Work out the finished part from the listing and answer in its coordinate system (mm). Coordinates: 2 decimals unless noted, no trailing zeros. Order: outer loops, then holes, each group sorted by start corner. A loop starts at its lowest first (then second) coordinate and runs counter-clockwise, first axis right, second up. Notation, with made-up numbers: M -39,82 L -30,82 A19 cw -30,95 Z; hole C 74.5,-27 d3. An arc over 180 degrees is marked long. Answer in a Markdown table with one row per item. Add a question column.
Item 1: Consider line 1 (X direction, y = 0.75, z = 0); line 2 (X direction, y = 1.3, z = -3); line 3 (Z direction, x = 82.55, y = 1.25). Determine where each line is inside the solid, lowest interval first. Write a range as from..to.
Item 2: The part is cut by section A-A (z = 0). Write down the section's boundary in (x, y).
Item 3: The part is cut by section D-D (x = 0). Write down the section's boundary in (y, z), then the cut area to 3 significant figures.
Item 4: The part is cut by section B-B (x = -88.9). Write down the section's boundary in (y, z).
Item 5: The part is cut by section C-C (y = 0.95). Write down the section's boundary in (x, z), then the cut area to 3 significant figures.
Item 6: A flat-ended cylindrical pin translates along its axis: pin 1 Ø5 at (x, z) = (0, 0) entering from +Y. Find the tip coordinate at first contact, or state that the pin passes through.
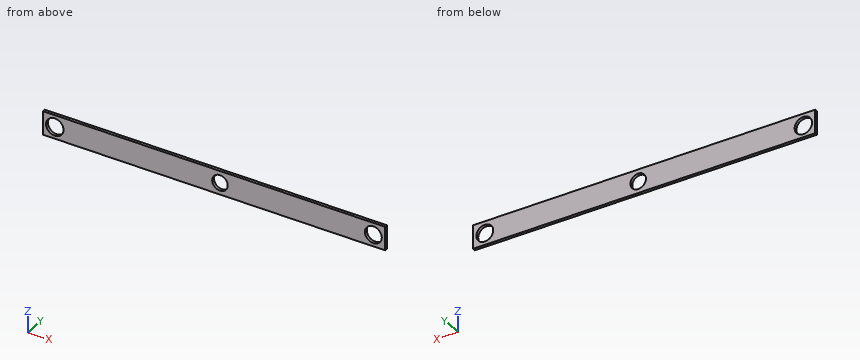
from build123d import *

# Parameters (mm, degrees)
SKETCH2_W           = 184.15
SKETCH2_H           = 12.7
SKETCH2_R           = 4.181180969
SKETCH2_R_2         = 4.536454583
SKETCH2_R_3         = 4.688788017
BOSS_EXTRUDE1_DEPTH = 1.5875


with BuildPart() as part:
    # Sketch2 → Boss-Extrude1 (new body)
    with BuildSketch(Plane(origin=(0, 0, 0), x_dir=(1, 0, 0), z_dir=(0, 1, 0))):
        with Locations((-3.175, -0.059345794)):
            Rectangle(SKETCH2_W, SKETCH2_H)
        Circle(SKETCH2_R, mode=Mode.SUBTRACT)
        with Locations((82.55, 0)):
            Circle(SKETCH2_R_2, mode=Mode.SUBTRACT)
        with Locations((-88.9, 0)):
            Circle(SKETCH2_R_3, mode=Mode.SUBTRACT)
    extrude(amount=BOSS_EXTRUDE1_DEPTH)


solid = part.part
Reply:
| question | item | result |
|---|---|---|
| 1 | line 1 | x = -95.25..-93.59, -84.21..-4.18, 4.18..78.01, 87.09..88.9 |
| 1 | line 2 | x = -95.25..-92.5, -85.3..-2.91, 2.91..79.15, 85.95..88.9 |
| 1 | line 3 | z = -6.29..-4.54, 4.54..6.41 |
| 2 | outline | M -95.25,0 L -93.59,0 L -93.59,1.59 L -95.25,1.59 Z; M -84.21,0 L -4.18,0 L -4.18,1.59 L -84.21,1.59 Z; M 4.18,0 L 78.01,0 L 78.01,1.59 L 4.18,1.59 Z; M 87.09,0 L 88.9,0 L 88.9,1.59 L 87.09,1.59 Z |
| 3 | outline | M 0,-6.29 L 1.59,-6.29 L 1.59,-4.18 L 0,-4.18 Z; M 0,4.18 L 1.59,4.18 L 1.59,6.41 L 0,6.41 Z |
| 3 | area | 6.89 mm2 |
| 4 | outline | M 0,-6.29 L 1.59,-6.29 L 1.59,-4.69 L 0,-4.69 Z; M 0,4.69 L 1.59,4.69 L 1.59,6.41 L 0,6.41 Z |
| 5 | outline | M -95.25,-6.29 L 88.9,-6.29 L 88.9,6.41 L -95.25,6.41 Z; hole C -88.9,0 d9.38; hole C 0,0 d8.36; hole C 82.55,0 d9.07 |
| 5 | area | 2,150 mm2 |
| 6 | pin 1 | passes through |
